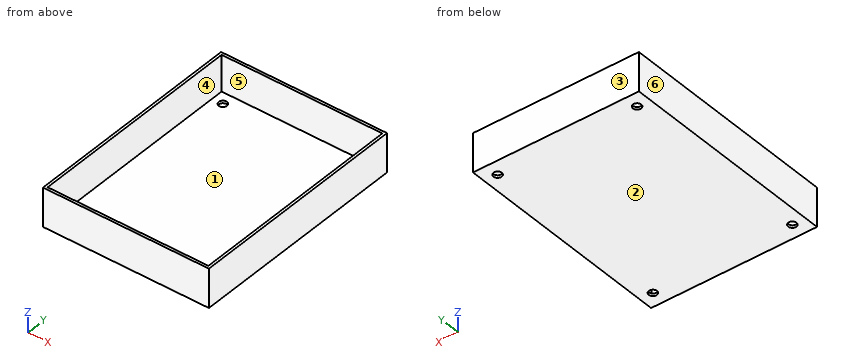
from build123d import *

# Parameters (mm, degrees)
SKETCH_1_W          = 64.2
SKETCH_1_H          = 86
EXTRUDE_1_DEPTH     = 15
SKETCH_2_W          = 62.2
SKETCH_2_H          = 84
CUT_EXTRUDE_1_DEPTH = 14
SKETCH_4_R          = 1.6
CUT_EXTRUDE_2_DEPTH = 1


with BuildPart() as part:
    # Эскиз1 → Бобышка-Вытянуть1 (new body)
    with BuildSketch(Plane.XY):
        Rectangle(SKETCH_1_W, SKETCH_1_H)
    extrude(amount=EXTRUDE_1_DEPTH)

    # Эскиз2 → Вырез-Вытянуть1 (cut)
    with BuildSketch(Plane.XY.offset(15)):
        Rectangle(SKETCH_2_W, SKETCH_2_H)
    extrude(amount=-CUT_EXTRUDE_1_DEPTH, mode=Mode.SUBTRACT)

    # Эскиз4 → Вырез-Вытянуть2 (cut)
    with BuildSketch(Plane(origin=(0, 0, 0), x_dir=(-1, 0, 0), z_dir=(0, 0, -1))):
        with Locations((-27, 37.5)):
            Circle(SKETCH_4_R)
        with Locations((27, 37.5)):
            Circle(SKETCH_4_R)
        with Locations((-27, -37.5)):
            Circle(SKETCH_4_R)
        with Locations((27, -37.5)):
            Circle(SKETCH_4_R)
    extrude(amount=-CUT_EXTRUDE_2_DEPTH, mode=Mode.SUBTRACT)


solid = part.part
CAD build for the part. Positions are in the model's coordinates, mm. Face numbers are marked on the shaded views. A direction names the side the tool comes from. Round coordinates to 2 decimals unless told otherwise and drop trailing zeros. Loops run counter-clockwise (first coordinate to the right, second up) from the corner with the lowest first, then second, coordinate; pieces in that order, holes last. Notation, with made-up numbers: M -25.75,65 L 33.25,65 A12 ccw 33.25,83 Z; hole C 1,79.25 d1. An arc over 180 degrees is marked long. One line per question, with ' | ' between items. Start each with the question number.
Item 1: Wall check: line 1 (Y direction, x = -27, z = 0.6); line 2 (X direction, y = -21, z = 5.5); line 3 (Y direction, x = -10.5, z = 11). Give the ranges that are in metal, low to high.
Item 2: Cut at A-A, the plane x = 27. Write the cut outline in (y, z), plus the area to 3 significant figures.
Item 3: Cut at C-C, the plane z = 8. Write the cut outline in (x, y).
Item 4: Cut at B-B, the plane y = 37.5. Write the cut outline in (x, z), plus the area to 3 significant figures.
Item 5: Two-plate mould, pull along X, no slides. Class the marked faces 3, 4, 5 and 6: pulls with the +X half, pulls with the -X half, needs draft (parallel to the pull), parting line crosses it, or undercut.
Item 6: Pin check, flat tip, straight feed: pin 1 Ø5 at (x, y) = (27, 37.5) entering from +Z. Stop position of the tip, or through.
Item 7: Cut at D-D, the plane x = -2.5. Write the cut outline in (y, z), plus the area to 3 significant figures.
Item 8: Which spindle directions (+Z, -Z, +X, -X, +Y, -Y) get a long thin tool onto all of the face, cutting with end or side? Do the marked faces 1 and 2. Say none if no direction does.
Responses:
1) line 1: y = -43 to -39.1, -35.9 to 35.9, 39.1 to 43 | line 2: x = -32.1 to -31.1, 31.1 to 32.1 | line 3: y = -43 to -42, 42 to 43
2) outline: M -43,0 L -39.1,0 L -39.1,1 L -42,1 L -42,15 L -43,15 Z; M -35.9,0 L 35.9,0 L 35.9,1 L -35.9,1 Z; M 39.1,0 L 43,0 L 43,15 L 42,15 L 42,1 L 39.1,1 Z | area: 108 mm²
3) outline: M -32.1,-43 L 32.1,-43 L 32.1,43 L -32.1,43 Z; hole M -31.1,-42 L 31.1,-42 L 31.1,42 L -31.1,42 Z
4) outline: M -32.1,0 L -28.6,0 L -28.6,1 L -31.1,1 L -31.1,15 L -32.1,15 Z; M -25.4,0 L 25.4,0 L 25.4,1 L -25.4,1 Z; M 28.6,0 L 32.1,0 L 32.1,15 L 31.1,15 L 31.1,1 L 28.6,1 Z | area: 85.8 mm²
5) face 3: needs draft | face 4: undercut | face 5: undercut | face 6: pulls with the -X half
6) pin 1: stops at z = 1
7) outline: M -43,0 L 43,0 L 43,15 L 42,15 L 42,1 L -42,1 L -42,15 L -43,15 Z | area: 114 mm²
8) face 1: +Z | face 2: -Z, +X, -X, +Y, -Y
